The model under review builds one solid part; all positions refer to its coordinate system, in mm. Face numbers are marked on the shaded views. A direction names the side the tool comes from. Round coordinates to 2 decimals unless told otherwise and drop trailing zeros. Order: outer loops, then holes, each group sorted by start corner. A loop starts at its lowest first (then second) coordinate and runs counter-clockwise, first axis right, second up. Notation, with made-up numbers: (87.5, 36.5) -> (114.5, 36.5) arc R11 ccw to (114.5, 43.5) -> close; hole circle Ø3 at (-23.75, -39). An arc over 180 degrees is marked (long way). Return JSON: item names as keys, results as strings. Group by question number.
from build123d import *

# Parameters (mm, degrees)
BOSS_EXTRUDE1_DEPTH     = 50
FILLET2_R               = 20
SKETCH6_R               = 1.5
CUT_EXTRUDE2_DEPTH      = 28.4
CUT_EXTRUDE3_DEPTH      = 136.4
CUT_EXTRUDE4_DEPTH      = 116.893533958
CUT_EXTRUDE4_DEPTH_BACK = 26.4


with BuildPart() as part:
    # Sketch1 → Boss-Extrude1 (new body)
    with BuildSketch(Plane(origin=(0, 0, 0), x_dir=(1, 0, 0), z_dir=(0, 1, 0))):
        with BuildLine():
            Line((-56.375697839, 54.197981352), (-56.375697839, 10.497981352))
            ThreePointArc((-56.375697839, 10.497981352), (-53.44676565, 3.42691354), (-46.375697839, 0.497981352))
            Line((-46.375697839, 0.497981352), (16.224302161, 0.497981352))
            ThreePointArc((16.224302161, 0.497981352), (23.295369973, 3.42691354), (26.224302161, 10.497981352))
            Line((26.224302161, 10.497981352), (26.224302161, 64.097981352))
            Line((26.224302161, 64.097981352), (19.224302161, 64.097981352))
            Line((19.224302161, 64.097981352), (19.224302161, 10.497981352))
            ThreePointArc((19.224302161, 10.497981352), (18.345622505, 8.376661008), (16.224302161, 7.497981352))
            Line((16.224302161, 7.497981352), (-46.375697839, 7.497981352))
            ThreePointArc((-46.375697839, 7.497981352), (-48.497018182, 8.376661008), (-49.375697839, 10.497981352))
            Line((-49.375697839, 10.497981352), (-49.375697839, 54.197981352))
            Line((-49.375697839, 54.197981352), (-56.375697839, 54.197981352))
        make_face()
    extrude(amount=BOSS_EXTRUDE1_DEPTH)

    # Fillet2
    fillet2_edges = [part.edges().sort_by_distance(p)[0] for p in [
        (22.724302161, 0, -64.097981352),
        (-52.875697839, 0, -54.197981352),
        (22.724302161, 50, -64.097981352),
        (-52.875697839, 50, -54.197981352),
    ]]
    fillet(fillet2_edges, radius=FILLET2_R)

    # Sketch6 → Cut-Extrude2 (cut)
    with BuildSketch(Plane(origin=(26.224302161, 0, 0), x_dir=(0, 0, -1), z_dir=(1, 0, 0))):
        with BuildLine():
            ThreePointArc((34.097981352, 25), (38.097981352, 21), (42.097981352, 25))
            Line((42.097981352, 25), (34.097981352, 25))
        make_face()
        with BuildLine():
            Line((34.097981352, 25), (42.097981352, 25))
            ThreePointArc((42.097981352, 25), (38.097981352, 29), (34.097981352, 25))
        make_face()
        with BuildLine():
            ThreePointArc((31.836343923, 25), (38.097981352, 18.738362572), (44.35961878, 25))
            Line((44.35961878, 25), (42.097981352, 25))
            ThreePointArc((42.097981352, 25), (38.097981352, 21), (34.097981352, 25))
            Line((34.097981352, 25), (31.836343923, 25))
        make_face()
        with BuildLine():
            Line((42.097981352, 25), (44.35961878, 25))
            ThreePointArc((44.35961878, 25), (38.097981352, 31.261637428), (31.836343923, 25))
            Line((31.836343923, 25), (34.097981352, 25))
            ThreePointArc((34.097981352, 25), (38.097981352, 29), (42.097981352, 25))
        make_face()
        with Locations((30.390517437, 32.707463915)):
            Circle(SKETCH6_R)
        with Locations((26.876196734, 36.221784617)):
            Circle(SKETCH6_R)
        with Locations((23.354804964, 39.743176388)):
            Circle(SKETCH6_R)
        with Locations((19.854626397, 43.243354955)):
            Circle(SKETCH6_R)
        with Locations((44.108388992, 31.01040764)):
            Circle(SKETCH6_R)
        with Locations((47.643922898, 34.545941546)):
            Circle(SKETCH6_R)
        with Locations((51.179456803, 38.081475452)):
            Circle(SKETCH6_R)
        with Locations((54.714990709, 41.617009358)):
            Circle(SKETCH6_R)
        with Locations((45.805445266, 17.292536085)):
            Circle(SKETCH6_R)
        with Locations((49.319765969, 13.778215383)):
            Circle(SKETCH6_R)
        with Locations((52.841157739, 10.256823612)):
            Circle(SKETCH6_R)
        with Locations((56.341336306, 6.756645045)):
            Circle(SKETCH6_R)
        with Locations((32.087573711, 18.98959236)):
            Circle(SKETCH6_R)
        with Locations((28.552039805, 15.454058454)):
            Circle(SKETCH6_R)
        with Locations((25.0165059, 11.918524548)):
            Circle(SKETCH6_R)
        with Locations((21.480971994, 8.382990642)):
            Circle(SKETCH6_R)
    extrude(amount=-CUT_EXTRUDE2_DEPTH, mode=Mode.SUBTRACT)

    # Sketch6_3 → Cut-Extrude3 (cut)
    with BuildSketch(Plane(origin=(26.224302161, 0, 0), x_dir=(0, 0, -1), z_dir=(1, 0, 0))):
        with BuildLine():
            ThreePointArc((34.097981352, 25), (38.097981352, 21), (42.097981352, 25))
            Line((42.097981352, 25), (34.097981352, 25))
        make_face()
        with BuildLine():
            Line((34.097981352, 25), (42.097981352, 25))
            ThreePointArc((42.097981352, 25), (38.097981352, 29), (34.097981352, 25))
        make_face()
    extrude(amount=-CUT_EXTRUDE3_DEPTH, mode=Mode.SUBTRACT)

    # Sketch7 → Cut-Extrude4 (cut, two sides: drawn at the far end of the back side and taken through both)
    with BuildSketch(Plane(origin=(26.224302161, 0, 0), x_dir=(0, 0, -1), z_dir=(1, 0, 0)).offset(-CUT_EXTRUDE4_DEPTH_BACK)):
        with BuildLine():
            Line((44.097981352, 50), (27.901409821, 50))
            Line((27.901409821, 50), (34.889942889, 40.363586132))
            ThreePointArc((34.889942889, 40.363586132), (38.136702541, 38.542544558), (41.629478365, 39.830239282))
            Line((41.629478365, 39.830239282), (48.26230961, 49.561655609))
            ThreePointArc((48.26230961, 49.561655609), (46.191648926, 49.890112018), (44.097981352, 50))
        make_face()
    extrude(amount=CUT_EXTRUDE4_DEPTH + CUT_EXTRUDE4_DEPTH_BACK, mode=Mode.SUBTRACT)


solid = part.part
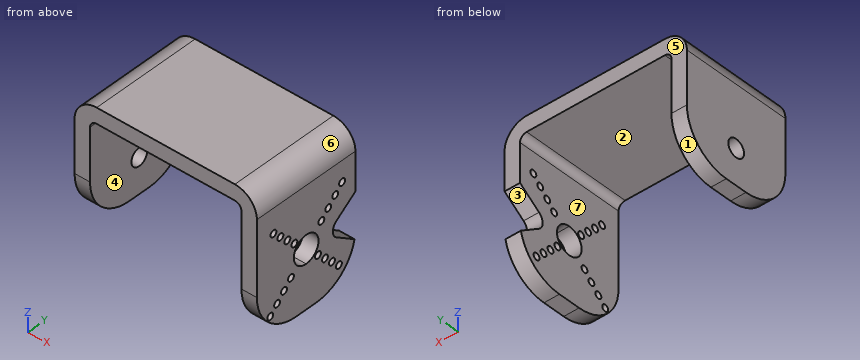
Item 1: Consider section A-A on z = -12.5. State the section outline as (x, y) points.
Item 2: Consider section B-B on x = -41.5. State the section outline as (y, z) points, plus the area to 3 significant figures.
Item 3: The part is to be moulded in two halves that separate along X. For the marked faces 4, 5, 6 and 7, say which applies: +X half, -X half, draft (parallel to the pull), parting line (faces both ways), or undercut.
Item 4: Wall thickness on line 1 along X through (y, z) = (37, -50); line 2 along Z through (x, y) = (11, 28); line 3 along X through (y, z) = (35.5, -54.5): over which ranges is each line inside the solid? List them lowest first.
Item 5: Consider section C-C on z = -36. State the section outline as (x, y) points.
Item 6: Insertion check: pin 1 Ø1.8 at (y, z) = (43.24, -19.85) entering from +X; pin 2 Ø5 at (x, y) = (-42.5, 33) entering from -Z; pin 3 Ø2 at (x, y) = (-51, 23) entering from -Z. Each pin has a flat end and moves straight along its axis. Give the tip position at first contact, or say it passes through.
Item 7: For the marked faces 1, 2 and 3, list the 3-axis set-ups (+Z, -Z, +X, -X, +Y, -Y) from which the entire face can be reached by the end or side of a thin tool; tool diameter is ignored.
Values:
{
 "1": {"outline": "(-56.38, 0) -> (-49.38, 0) -> (-49.38, 50) -> (-56.38, 50) -> close; (19.22, 0) -> (26.22, 0) -> (26.22, 50) -> (19.22, 50) -> close"},
 "2": {"outline": "(0, -7.5) -> (50, -7.5) -> (50, -0.5) -> (0, -0.5) -> close", "area": "350 mm^2"},
 "3": {"face 4": "undercut", "face 5": "draft", "face 6": "+X half", "face 7": "undercut"},
 "4": {"line 1": "-56.38 to -49.38, 19.22 to 26.22", "line 2": "-7.5 to -0.5", "line 3": "19.22 to 26.22"},
 "5": {"outline": "(-56.38, 0.08) -> (-49.38, 0.08) -> (-49.38, 21.59) -> (-56.38, 21.59) -> close; (-56.38, 28.41) -> (-49.38, 28.41) -> (-49.38, 49.92) -> (-56.38, 49.92) -> close; (19.22, 0) -> (26.22, 0) -> (26.22, 19.1) -> (19.22, 19.1) -> close; (19.22, 30.9) -> (26.22, 30.9) -> (26.22, 39.29) -> (19.22, 39.29) -> close"},
 "6": {"pin 1": "x = -49.38", "pin 2": "z = -7.5", "pin 3": "z = -54.2"},
 "7": {"face 1": "-Z, -X, +Y", "face 2": "-Z, +Y, -Y", "face 3": "+X, +Y"}
}
